from build123d import *

# Parameters (mm, degrees)
SKETCH_1_W          = 50
SKETCH_1_H          = 19.4
EXTRUDE_1_DEPTH     = 3
SKETCH_2_W          = 18.05
SKETCH_2_H          = 3
SKETCH_2_W_2        = 9.27
EXTRUDE_3_DEPTH     = 12
SKETCH_5_R          = 1
CUT_EXTRUDE_1_DEPTH = 4
SKETCH_6_W          = 9.27
SKETCH_6_H          = 2.996679997
EXTRUDE_5_DEPTH     = 21
SKETCH_9_W          = 7.5
SKETCH_9_H          = 2.996679997
EXTRUDE_6_DEPTH     = 5
SKETCH_10_W         = 7.5
SKETCH_10_H         = 2.996679997
EXTRUDE_7_DEPTH     = 5
SKETCH_11_R         = 2.15
SKETCH_11_R_2       = 1.65
CUT_EXTRUDE_3_DEPTH = 5
SKETCH_12_R         = 2
SKETCH_12_R_2       = 1.65
CUT_EXTRUDE_4_DEPTH = 5


with BuildPart() as part:
    # 草图1 → 凸台-拉伸1 (new body)
    with BuildSketch(Plane.XY):
        with Locations((25, 9.7)):
            Rectangle(SKETCH_1_W, SKETCH_1_H)
    extrude(amount=EXTRUDE_1_DEPTH)

    # 草图2 → 凸台-拉伸3 (add)
    with BuildSketch(Plane(origin=(0, 0, 0), x_dir=(-1, 0, 0), z_dir=(0, 0, -1))):
        with Locations((-40.975, 17.9)):
            Rectangle(SKETCH_2_W, SKETCH_2_H)
        with Locations((-4.635, 17.9)):
            Rectangle(SKETCH_2_W_2, SKETCH_2_H)
    extrude(amount=EXTRUDE_3_DEPTH)

    # 草图5 → 切除-拉伸1 (cut)
    with BuildSketch(Plane(origin=(0, 19.4, 0), x_dir=(1, 0, 0), z_dir=(0, 1, 0))):
        with Locations((34.45, 6)):
            Circle(SKETCH_5_R)
        with Locations((6.78, 6)):
            Circle(SKETCH_5_R)
    extrude(amount=-CUT_EXTRUDE_1_DEPTH, mode=Mode.SUBTRACT)

    # 草图6 → 凸台-拉伸5 (add)
    with BuildSketch(Plane(origin=(0, 0, 0), x_dir=(-1, 0, 0), z_dir=(0, 0, -1))):
        with Locations((-45.365, 1.498339999)):
            Rectangle(SKETCH_6_W, SKETCH_6_H)
        with Locations((-4.635, 1.498339999)):
            Rectangle(SKETCH_6_W, SKETCH_6_H)
    extrude(amount=EXTRUDE_5_DEPTH)

    # 草图9 → 凸台-拉伸6 (add)
    with BuildSketch(Plane(origin=(9.27, 0, 0), x_dir=(0, 0, -1), z_dir=(1, 0, 0))):
        with Locations((17.25, 1.498339999)):
            Rectangle(SKETCH_9_W, SKETCH_9_H)
    extrude(amount=EXTRUDE_6_DEPTH)

    # 草图10 → 凸台-拉伸7 (add)
    with BuildSketch(Plane.ZY.offset(-40.73)):
        with Locations((-17.25, 1.498339999)):
            Rectangle(SKETCH_10_W, SKETCH_10_H)
    extrude(amount=EXTRUDE_7_DEPTH)

    # 草图11 → 切除-拉伸3 (cut)
    with BuildSketch(Plane(origin=(0, 2.996679997, 0), x_dir=(1, 0, 0), z_dir=(0, 1, 0))):
        with Locations((42.5, 16.75)):
            Circle(SKETCH_11_R)
        with Locations((46.5, 3.5)):
            Circle(SKETCH_11_R_2)
    extrude(amount=-CUT_EXTRUDE_3_DEPTH, mode=Mode.SUBTRACT)

    # 草图12 → 切除-拉伸4 (cut)
    with BuildSketch(Plane(origin=(0, 2.996679997, 0), x_dir=(1, 0, 0), z_dir=(0, 1, 0))):
        with Locations((7.5, 16.75)):
            Circle(SKETCH_12_R)
        with Locations((3.5, 3.5)):
            Circle(SKETCH_12_R_2)
    extrude(amount=-CUT_EXTRUDE_4_DEPTH, mode=Mode.SUBTRACT)


solid = part.part
The model under review builds one solid part; all positions refer to its coordinate system, in mm. A direction names the side the tool comes from. Give positions to 0.01 mm unless a question says otherwise; leave off trailing zeros. Loops run counter-clockwise (first coordinate to the right, second up) from the corner with the lowest first, then second, coordinate; pieces in that order, holes last. Notation, with made-up numbers: (1, -16.75) -> (23, -16.75) arc R27 ccw to (23, 13.25) -> close; hole circle Ø9 at (81.25, 11). An arc over 180 degrees is marked (long way). Put each result on its own line as item: value. Start each with the question number.
1. Clearance check with flat-ended pins moving along their axes: P1, Ø2, axis at x = 39.5, y = 6.5, coming from the -Z side; P2, Ø3.5, axis at x = 42.5, z = -16.75, coming from the -Y side; P3, Ø3, axis at x = 46.5, z = -3.5, coming from the -Y side. State where each tip first meets the part, or that it passes through.
2. We need section B-B on y = 18. State the section outline as (x, z) points.
3. For faces 4 (the face through (5, 2.997, -10)), 5 (the face through (40.73, 1, -7)), 6 (the face through (5, 18, -12)), 7 (the face through (31.95, 18, -6)), 8 (the face through (6.65, 17.92, -6.99)), list the 3-axis set-ups (+Z, -Z, +X, -X, +Y, -Y) from which the entire face can be reached by the end or side of a thin tool; tool diameter is ignored.
4. Mouldability with a two-part tool opening along Z and no side actions: class faces 1 (the face through (14.27, 2, -17)), 2 (the face through (25, 10, 3)), 3 (the face through (38, 1, -13.5)) as released by +Z, released by -Z, zero draft, split by the parting line, or undercut.
5. We need section A-A on x = 37.5. State the section outline as (y, z) points.
6. We need section D-D on z = -16.75. State the section outline as (x, y) points, then the cut area to 3 significant figures.
7. Wall thickness on probe 1 along X at (y, z) = (0.75, -16.75); probe 2 along Z at (x, y) = (7.5, 2.35); probe 3 along X at (y, z) = (18.4, -6): over which ranges is each line inside the solid? List them lowest first.
8. We need section C-C on z = -3.5. State the section outline as (x, y) points, then the cut area to 3 significant figures.
Determined:
1. P1: z = 0
1. P2: through
1. P3: y = 16.4
2. outline: (0, -12) -> (9.27, -12) -> (9.27, 0) -> (31.95, 0) -> (31.95, -12) -> (50, -12) -> (50, 3) -> (0, 3) -> close; hole circle Ø2 at (6.78, -6); hole circle Ø2 at (34.45, -6)
3. face 4: -Z, +X, -X
3. face 5: -Y
3. face 6: -Z, +X, -X, +Y
3. face 7: -Z, +Y, -Y
3. face 8: +Y
4. face 1: zero draft
4. face 2: released by +Z
4. face 3: undercut
5. outline: (0, -21) -> (3, -21) -> (3, -13.5) -> (0, -13.5) -> close; (0, 0) -> (16.4, 0) -> (16.4, -12) -> (19.4, -12) -> (19.4, 3) -> (0, 3) -> close
6. outline: (0, 0) -> (5.5, 0) -> (5.5, 3) -> (0, 3) -> close; (9.5, 0) -> (14.27, 0) -> (14.27, 3) -> (9.5, 3) -> close; (35.73, 0) -> (40.35, 0) -> (40.35, 3) -> (35.73, 3) -> close; (44.65, 0) -> (50, 0) -> (50, 3) -> (44.65, 3) -> close
6. area: 60.7 mm^2
7. probe 1: 0 to 5.5, 9.5 to 14.27, 35.73 to 40.35, 44.65 to 50
7. probe 2: -21 to -18.75, -14.75 to 3
7. probe 3: 0 to 5.78, 7.78 to 9.27, 31.95 to 33.45, 35.45 to 50
8. outline: (0, 0) -> (1.85, 0) -> (1.85, 3) -> (0, 3) -> close; (0, 16.4) -> (9.27, 16.4) -> (9.27, 19.4) -> (0, 19.4) -> close; (5.15, 0) -> (9.27, 0) -> (9.27, 3) -> (5.15, 3) -> close; (31.95, 16.4) -> (50, 16.4) -> (50, 19.4) -> (31.95, 19.4) -> close; (40.73, 0) -> (44.85, 0) -> (44.85, 3) -> (40.73, 3) -> close; (48.15, 0) -> (50, 0) -> (50, 3) -> (48.15, 3) -> close
8. area: 118 mm^2
